The model under review builds one solid part; all positions refer to its coordinate system, in mm. Face numbers are marked on the shaded views. A direction names the side the tool comes from. Round coordinates to 2 decimals unless told otherwise and drop trailing zeros. Write each loop counter-clockwise with the first axis right and the second up, starting at its lowest first coordinate (ties: lowest second). Pieces come first, ordered by that corner, then holes. Notation, with made-up numbers: (34, 9) - (73, 9) arc R16 cw to (73, 31) - close; hole circle Ø7 at (42.25, 54.5). An arc over 180 degrees is marked (long way). One line per question, with ' | ' between items. Start each with the question number.
```python
from build123d import *

# Parameters (mm, degrees)
F1_DEPTH  = 25
F2_W      = 62
F2_H      = 83
F3_DEPTH  = 18
F4_W      = 46
F4_H      = 83
F5_DEPTH  = 5
F7_D      = 2.5
F7_DEPTH  = 5.5
F7_TIP    = 0.7510757738
F8_W      = 62
F8_H      = 15
F9_DEPTH  = 25.001
F11_D     = 8
F12_W     = 6
F12_H     = 16.5
F12_H_2   = 13.5
F12_W_2   = 7
F13_DEPTH = 1.5
F14_W     = 8
F14_H     = 18
F15_DEPTH = 2
F16_R     = 4.25
F17_DEPTH = 1.5
F18_W     = 5
F18_H     = 0.7
F19_DEPTH = 5
F21_D     = 2.5
F21_DEPTH = 7
F21_TIP   = 0.7510757738


# Not quite as in the source:
# - a pattern or mirror of a feature is missing from the dataset's text; its kind, count and spacing are read off the source's solid


with BuildPart() as f1:
    # F0 (on Top) → F1 (new body)
    with BuildSketch(Plane.XY):
        Polygon((40, 48), (-40, 48), (-40, -38), (-57.5, -38), (-57.5, -48), (57.5, -48), (57.5, -38), (40, -38), align=None)
    extrude(amount=F1_DEPTH)

    # F2 (on face) → F3 (cut)
    with BuildSketch(Plane.XY.offset(25)):
        with Locations((0, 5)):
            Rectangle(F2_W, F2_H)
    extrude(amount=-F3_DEPTH, mode=Mode.SUBTRACT)

    # F4 (on face) → F5 (cut)
    with BuildSketch(Plane.XY.offset(7)):
        with Locations((0, 5)):
            Rectangle(F4_W, F4_H)
    extrude(amount=-F5_DEPTH, mode=Mode.SUBTRACT)

    # F7
    with Locations(Plane.XY.offset(7)):
        with Locations((-27, -32.5), (-27, -2.5), (-27, 23.5), (27, -32.5), (27, -2.5), (27, 23.5)):
            Hole(F7_D / 2, depth=F7_DEPTH)
            with Locations((0, 0, -(F7_DEPTH + F7_TIP / 2))):  # 118° drill point
                Cone(0, F7_D / 2, F7_TIP, mode=Mode.SUBTRACT)

    # F8 (on face) → F9 (cut, through all)
    with BuildSketch(Plane(origin=(0, 0, 0), x_dir=(1, 0, 0), z_dir=(0, 0, -1))):
        with Locations((0, 17.5)):
            Rectangle(F8_W, F8_H)
    extrude(amount=-F9_DEPTH, mode=Mode.SUBTRACT)

    # F11 (through all)
    with Locations(Plane(origin=(0, -38, 0), x_dir=(-1, 0, 0), z_dir=(0, 1, 0))):
        with Locations((50.8, 12.5), (-50.8, 12.5)):
            Hole(F11_D / 2)

    # F12 (on face) → F13 (cut, through all)
    with BuildSketch(Plane(origin=(0, 48, 0), x_dir=(-1, 0, 0), z_dir=(0, 1, 0))):
        with Locations((-2, 16.75)):
            Rectangle(F12_W, F12_H)
        with Locations((11, 18.25)):
            Rectangle(F12_W, F12_H_2)
        with Locations((23, 16.75)):
            Rectangle(F12_W_2, F12_H)
    extrude(amount=-F13_DEPTH, mode=Mode.SUBTRACT)

    # F14 (on face) → F15 (cut)
    with BuildSketch(Plane.XY.offset(7)):
        with Locations((-27, 37.5)):
            Rectangle(F14_W, F14_H)
    extrude(amount=-F15_DEPTH, mode=Mode.SUBTRACT)

    # F16 (on face) → F17 (cut, through all)
    with BuildSketch(Plane(origin=(0, 48, 0), x_dir=(-1, 0, 0), z_dir=(0, 1, 0))):
        with Locations((-25, 17)):
            Circle(F16_R)
    extrude(amount=-F17_DEPTH, mode=Mode.SUBTRACT)

    # F18 (on face) → F19 (cut)
    with BuildSketch(Plane.YZ.offset(40)):
        with Locations((-35.5, 0.35)):
            Rectangle(F18_W, F18_H)
    f19 = extrude(amount=-F19_DEPTH, mode=Mode.SUBTRACT)

    # F19_copies: F19 across plane
    add(f19.mirror(Plane(origin=(0, 0, 0), x_dir=(0, 0, -1), z_dir=(-1, 0, 0))), mode=Mode.SUBTRACT)

    # F21
    with Locations(Plane.XY.offset(25)):
        with Locations((25, -43), (-25, -43), (35.5, 27), (-35.5, 27)):
            Hole(F21_D / 2, depth=F21_DEPTH)
            with Locations((0, 0, -(F21_DEPTH + F21_TIP / 2))):  # 118° drill point
                Cone(0, F21_D / 2, F21_TIP, mode=Mode.SUBTRACT)


solid = f1.part
```
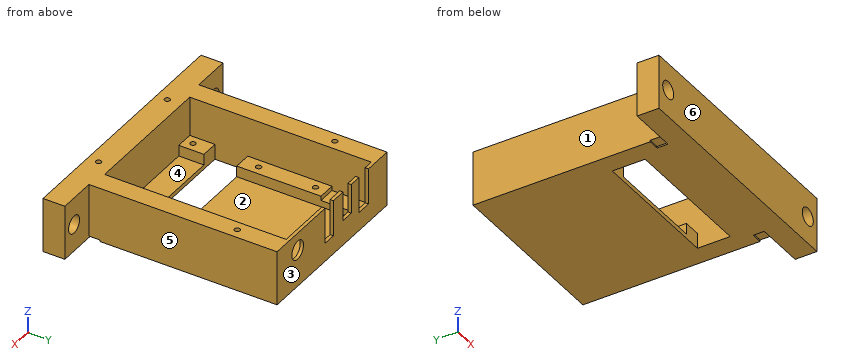
1. Wall thickness on line 1 along X through (y, z) = (-32.5, 5.15); line 2 along Y through (x, z) = (27, 3); line 3 along X through (y, z) = (-43, 20.25): over which ranges is each line inside the solid? List them lowest first. Write a range as [from, to].
2. Add section B-B, the plane x = 18.5. Write out the cut boundary in (y, z).
3. Clearance check with flat-ended pins moving along their axes: P1, Ø5, axis at y = -12, z = 3, coming from the -X side; P2, Ø23, axis at x = 4.5, y = 27.5, coming from the +Z side; P3, Ø2, axis at x = -35.5, y = 27, coming from the +Z side. State where each tip first meets the part, or that it passes through.
4. Add section A-A, the plane z = 3.25. Write out the cut boundary in (x, y).
5. Add section D-D, the plane x = -50.8. Write out the cut boundary in (y, z).
6. Machinability: for the marked faces 1, 2 and 3, which of the approach directions +Z, -Z, +X, -X, +Y, -Y give a long, thin tool a straight path to every point of the face, cutting with its end or side? Answer none if there is none.
7. Add section C-C, the plane y = 9.5. Write out the cut boundary in (x, z), then the cut area to 3 significant figures.
8. The part is to be moulded in two halves that separate along Y. For the marked faces 4, 5 and 6, say which applies: pulls with the +Y half, pulls with the -Y half, needs draft (parallel to the pull), parting line crosses it, or undercut.
Geometry check:
1) line 1: x = [-40, -28.25], [-25.75, -23], [23, 25.75], [28.25, 40] | line 2: y = [-48, -33.75], [-31.25, -25], [-10, -3.75], [-1.25, 22.25], [24.75, 48] | line 3: x = [-57.5, -26.25], [-23.75, 23.75], [26.25, 57.5]
2) outline: (-48, 0) - (-25, 0) - (-25, 2) - (-36.5, 2) - (-36.5, 25) - (-48, 25) - close; (-10, 0) - (48, 0) - (48, 25) - (46.5, 25) - (46.5, 2) - (-10, 2) - close
3) P1: stops at x = -40 | P2: stops at z = 2 | P3: stops at z = 17.85
4) outline: (-57.5, -48) - (57.5, -48) - (57.5, -38) - (40, -38) - (40, 48) - (-40, 48) - (-40, -38) - (-57.5, -38) - close; hole (-31, -25) - (-23, -25) - (-23, -36.5) - (23, -36.5) - (23, -25) - (31, -25) - (31, -10) - (23, -10) - (23, 46.5) - (-23, 46.5) - (-23, -10) - (-31, -10) - close; hole circle Ø2.5 at (-27, -32.5); hole circle Ø2.5 at (-27, -2.5); hole circle Ø2.5 at (-27, 23.5); hole circle Ø2.5 at (27, -32.5); hole circle Ø2.5 at (27, -2.5); hole circle Ø2.5 at (27, 23.5)
5) outline: (-48, 0) - (-38, 0) - (-38, 8.5) - (-48, 8.5) - close; (-48, 16.5) - (-38, 16.5) - (-38, 25) - (-48, 25) - close
6) face 1: +Z, -Z, -X, +Y | face 2: +Z | face 3: +Z, -Z, +X, -X, +Y
7) outline: (-40, 0) - (40, 0) - (40, 25) - (31, 25) - (31, 7) - (23, 7) - (23, 2) - (-23, 2) - (-23, 7) - (-31, 7) - (-31, 25) - (-40, 25) - close | area: 654 mm2
8) face 4: undercut | face 5: needs draft | face 6: pulls with the -Y half
